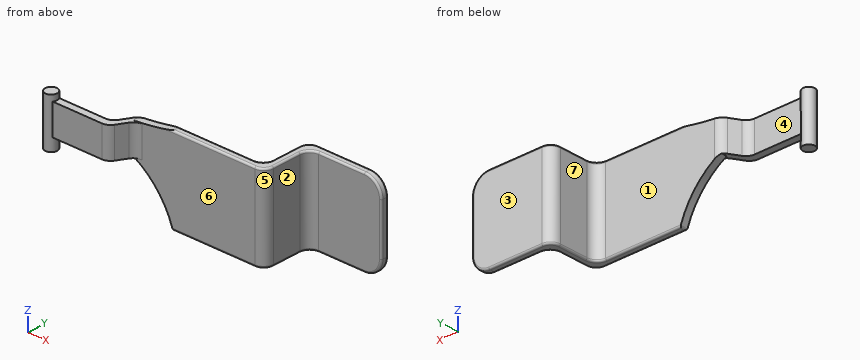
from build123d import *

# Parameters (mm, degrees)
SKETCH2_R            = 2.48
BOSS_EXTRUDE1_DEPTH  = 20
SKETCH3_W            = 24.73
SKETCH3_H            = 12.48
BOSS_EXTRUDE3_DEPTH  = 1.5
BOSS_EXTRUDE7_DEPTH  = 12.48
BOSS_EXTRUDE9_DEPTH  = 3
SKETCH9_W            = 10
SKETCH9_H            = 3
BOSS_EXTRUDE10_DEPTH = 34.71
SKETCH10_W           = 3
SKETCH10_H           = 23
BOSS_EXTRUDE11_DEPTH = 34.71
SKETCH11_W           = 34.71
SKETCH11_H           = 3
BOSS_EXTRUDE12_DEPTH = 30
FILLET1_R            = 4
FILLET3_R            = 7
FILLET4_R            = 0.75


with BuildPart() as part:
    # Sketch2 → Boss-Extrude1 (new body)
    with BuildSketch(Plane.XY):
        Circle(SKETCH2_R)
    extrude(amount=BOSS_EXTRUDE1_DEPTH)

    # Sketch3 → Boss-Extrude3 (add, symmetric)
    with BuildSketch(Plane(origin=(0, 0, 0), x_dir=(1, 0, 0), z_dir=(0, 1, 0))):
        with Locations((12.365, -11.34)):
            Rectangle(SKETCH3_W, SKETCH3_H)
    extrude(amount=BOSS_EXTRUDE3_DEPTH, both=True)

    # Sketch7 → Boss-Extrude7 (add)
    with BuildSketch(Plane.XY.offset(5.1)):
        Polygon((21.73, -1.5), (24.73, -1.5), (31.062035578, 9.5), (28.062035578, 9.5), align=None)
    extrude(amount=BOSS_EXTRUDE7_DEPTH)

    # Sketch8 → Boss-Extrude9 (add)
    with BuildSketch(Plane(origin=(0, 9.5, 0), x_dir=(1, 0, 0), z_dir=(0, 1, 0))):
        with BuildLine():
            Line((72.552035578, -20.06), (44.552035578, -20.06))
            ThreePointArc((44.552035578, -20.06), (36.356523667, -18.490944118), (28.062035578, -17.58))
            Line((28.062035578, -17.58), (28.062035578, -5.1))
            ThreePointArc((28.062035578, -5.1), (38.220194009, 3.177633796), (44.552035578, 14.65))
            Line((44.552035578, 14.65), (72.552035578, 14.65))
            Line((72.552035578, 14.65), (72.552035578, -20.06))
        make_face()
    extrude(amount=-BOSS_EXTRUDE9_DEPTH)

    # Sketch9 → Boss-Extrude10 (add)
    with BuildSketch(Plane.XY.offset(20.06)):
        with Locations((77.552035578, 8)):
            Rectangle(SKETCH9_W, SKETCH9_H)
    extrude(amount=-BOSS_EXTRUDE10_DEPTH)

    # Sketch10 → Boss-Extrude11 (add)
    with BuildSketch(Plane.XY.offset(20.06)):
        with Locations((81.052035578, 18)):
            Rectangle(SKETCH10_W, SKETCH10_H)
    extrude(amount=-BOSS_EXTRUDE11_DEPTH)

    # Sketch11 → Boss-Extrude12 (add)
    with BuildSketch(Plane(origin=(82.552035578, 0, 0), x_dir=(0, 0, -1), z_dir=(1, 0, 0))):
        with Locations((-2.705, 28)):
            Rectangle(SKETCH11_W, SKETCH11_H)
    extrude(amount=BOSS_EXTRUDE12_DEPTH)

    # Fillet1
    fillet1_edges = [part.edges().sort_by_distance(p)[0] for p in [
        (24.73, -1.5, 11.34),
        (82.552035578, 26.5, 2.705),
        (23.456918794, 1.5, 11.34),
        (28.062035578, 9.5, 11.34),
        (29.335116784, 6.5, 11.34),
        (82.552035578, 6.5, 2.705),
        (79.552035578, 9.5, 2.705),
        (79.552035578, 29.5, 2.705),
    ]]
    fillet(fillet1_edges, radius=FILLET1_R)

    # Fillet3
    fillet3_edges = [part.edges().sort_by_distance(p)[0] for p in [
        (112.552035578, 28, 20.06),
        (112.552035578, 28, -14.65),
    ]]
    fillet(fillet3_edges, radius=FILLET3_R)

    # Fillet4
    fillet4_edges = [part.edges().sort_by_distance(p)[0] for p in [
        (60.052035578, 9.5, -14.65),
        (61.552035578, 6.5, -14.65),
        (82.552035578, 16.5, 20.06),
        (79.552035578, 19.5, 20.06),
        (80.723608453, 28.328427125, 20.06),
        (81.380462702, 7.671572875, 20.06),
        (82.552035578, 16.5, -14.65),
        (79.552035578, 19.5, -14.65),
        (80.723608453, 28.328427125, -14.65),
        (81.380462702, 7.671572875, -14.65),
        (78.380462702, 10.671572875, -14.65),
        (78.380462702, 10.671572875, 20.06),
        (83.723608453, 25.328427125, -14.65),
        (83.723608453, 25.328427125, 20.06),
        (112.552035578, 26.5, 2.705),
        (112.552035578, 29.5, 2.705),
        (96.052035578, 26.5, 20.06),
        (96.052035578, 26.5, -14.65),
        (110.501783046, 26.5, -12.599747468),
        (110.501783046, 26.5, 18.009747468),
        (94.552035578, 29.5, 20.06),
        (94.552035578, 29.5, -14.65),
        (110.501783046, 29.5, -12.599747468),
        (110.501783046, 29.5, 18.009747468),
        (60.052035578, 9.5, 20.06),
        (44.552035578, 8, -14.65),
        (61.552035578, 6.5, 20.06),
    ]]
    fillet(fillet4_edges, radius=FILLET4_R)


with BuildPart() as body_2:
    # Mirror5: mirrored copy
    add(part.part.mirror(Plane(origin=(119.85106591, 0, 0), x_dir=(0, 0, 1), z_dir=(1, 0, 0))))


with BuildPart() as body_2_2:
    # Mirror6: mirrored copy
    add(body_2.part.mirror(Plane(origin=(119.85106591, 0, 0), x_dir=(0, 0, 1), z_dir=(1, 0, 0))))


solid = body_2_2.part
The listing builds one solid part. Answer for the finished solid, in the listing's coordinates (mm). Face numbers are marked on the shaded views. A direction names the side the tool comes from. Coordinates: 2 decimals unless noted, no trailing zeros. Write each loop counter-clockwise with the first axis right and the second up, starting at its lowest first coordinate (ties: lowest second). Pieces come first, ordered by that corner, then holes. Notation, with made-up numbers: M -0.5,6 L 48.5,6 A27 cw 48.5,40 Z; hole C -36,68 d10. An arc over 180 degrees is marked long. Write each question's results on one line, items separated by ' | '.
Item 1: Given P1, Ø1.5, axis at x = 12, z = 16, coming from the -Y side; P2, Ø6, axis at y = 16.5, z = 0, coming from the -X side; P3, Ø5, axis at x = 30, z = -2, coming from the +Y side; P4, Ø5, axis at x = 70.5, z = 11, coming from the -Y side, each flat-ended and moving along its own axis, determine where each tip first touches the part or whether it passes through.
Answer below:
P1: y = -1.5 | P2: x = 79.55 | P3: through | P4: y = 6.5
Item 2: The part is cut by section C-C on y = 18. Determine the outline of the cut face in (x, z), and give its area (3 significant figures).
Answer below:
outline: M 79.55,-13.9 A0.75 ccw 80.3,-14.65 L 81.8,-14.65 A0.75 ccw 82.55,-13.9 L 82.55,19.31 A0.75 ccw 81.8,20.06 L 80.3,20.06 A0.75 ccw 79.55,19.31 Z | area: 104 mm2
Item 3: Consider probe 1 along Y at (x, z) = (43, 7); probe 2 along Z at (x, y) = (17, 1); probe 3 along Y at (x, z) = (102, -6.5). Determine where each line is inside the solid, lowest interval first. Write a range as [from, to].
Answer below:
probe 1: [6.5, 9.5] | probe 2: [5.1, 17.58] | probe 3: [26.5, 29.5]
Item 4: The part is cut by section B-B on x = 55. Determine the outline of the cut face in (y, z), and give its area (3 significant figures).
Answer below:
outline: M 6.5,-13.9 A0.75 ccw 7.25,-14.65 L 8.75,-14.65 A0.75 ccw 9.5,-13.9 L 9.5,19.31 A0.75 ccw 8.75,20.06 L 7.25,20.06 A0.75 ccw 6.5,19.31 Z | area: 104 mm2
Item 5: The part is cut by section A-A on z = 11.5. Determine the outline of the cut face in (x, y).
Answer below:
outline: M 1.97,-1.5 L 22.42,-1.5 A4 ccw 25.88,0.5 L 28.18,4.5 A4 cw 31.65,6.5 L 78.55,6.5 A4 ccw 82.55,10.5 L 82.55,22.5 A4 cw 86.55,26.5 L 111.8,26.5 A0.75 ccw 112.55,27.25 L 112.55,28.75 A0.75 ccw 111.8,29.5 L 83.55,29.5 A4 ccw 79.55,25.5 L 79.55,13.5 A4 cw 75.55,9.5 L 30.37,9.5 A4 ccw 26.91,7.5 L 24.61,3.5 A4 cw 21.14,1.5 L 1.97,1.5 A2.48 ccw long Z
Item 6: For a pull along X with two mould halves and no side action, classify the marked faces 4, 5, 6 and 7 as released by +X, released by -X, zero draft, split by the parting line, or undercut.
Answer below:
face 4: undercut | face 5: released by +X | face 6: zero draft | face 7: released by -X
Item 7: The part is cut by section D-D on x = 0. Determine the outline of the cut face in (y, z).
Answer below:
outline: M -2.48,0 L 2.48,0 L 2.48,20 L -2.48,20 Z
Item 8: Which of the six approach directions +Z, -Z, +X, -X, +Y, -Y give full straight-line access (tool end or side, diameter ignored) to the marked faces 1, 2 and 3?
Answer below:
face 1: +Z, -Z, -X, +Y | face 2: +Z, -Z, +X, -Y | face 3: +Z, -Z, +X, -X, +Y
